Check sheet for the drawn part. Datum: minimum x, y, z corner. Units: mm. A direction names the side the tool comes from. Give positions to 0.01 mm unless a question says otherwise; leave off trailing zeros. Loops run counter-clockwise (first coordinate to the right, second up) from the corner with the lowest first, then second, coordinate; pieces in that order, holes last.
1. Cross-section at D-D, the plane x = 0.8. Record the cut outline in (y, z) (1 decimal).
2. Cross-section at B-B, the plane y = 6.75. Record the cut outline in (x, z) (1 decimal).
3. Tool access check on the marked faces 1, 2 and 3. Record the directions out of +Z, -Z, +X, -X, +Y, -Y that give a thin tool (end or side, any length) a straight path to the whole face; none if there is none.
4. Cross-section at C-C, the plane z = 13.75. Record the cut outline in (x, y).
5. Material ranges on L1, parallel to Z at x = 1.1, y = 11.5; L2, parallel to Z at x = 3.9, y = 12.25 (1 decimal); L3, parallel to Z at x = 1.2, y = 3, recorded low to high.
6. Go/stop test with flat-tipped pins: pin 1 Ø2 at (y, z) = (5, 9.5) entering from -X; pin 2 Ø1.7 at (y, z) = (2.159, 19.685) entering from -X; pin 3 Ø1.6 at (x, y) = (4, 9.5) entering from +Z (3 decimals); pin 4 Ø2.5 at (x, z) = (3.5, 11) entering from -Y. Record where each tip stops, or that it passes through.
7. Cross-section at A-A, the plane z = 2.5. Record the cut outline in (x, y) (1 decimal).
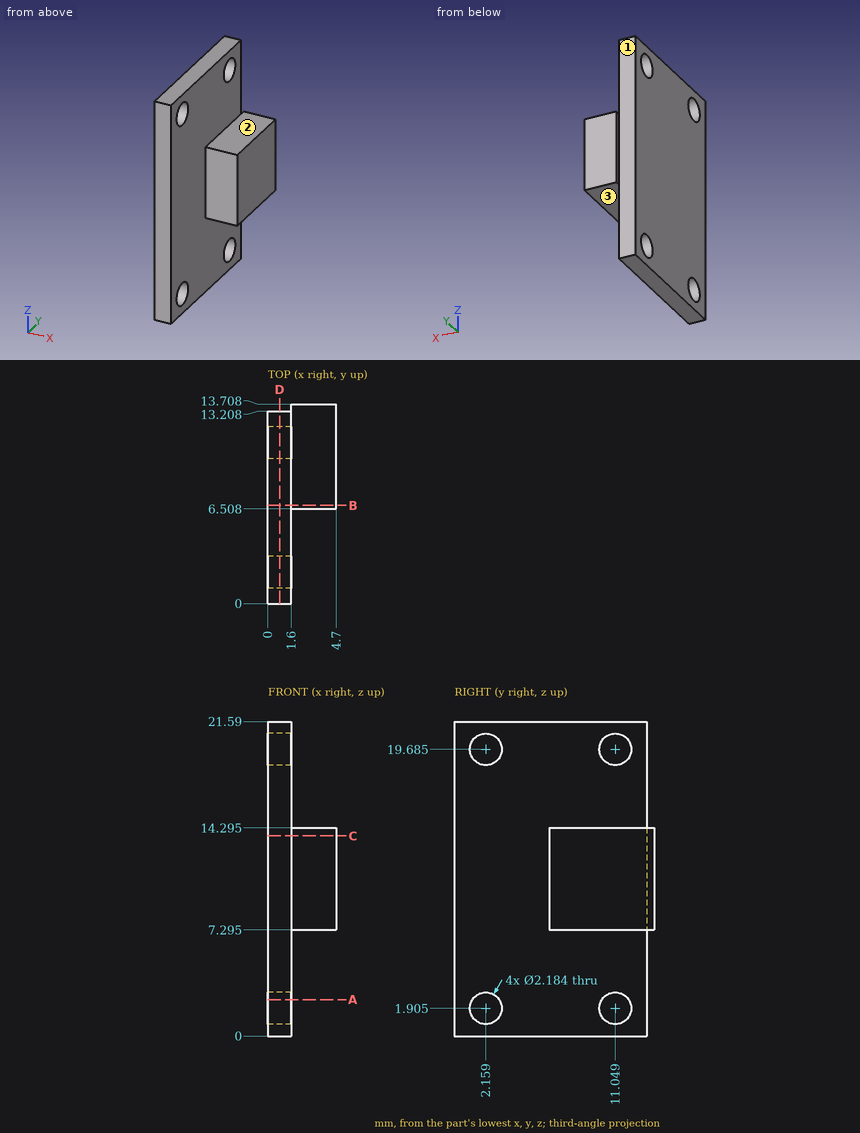
Result:
1. outline: (0, 0) - (13.2, 0) - (13.2, 21.6) - (0, 21.6) - close; hole circle Ø2.2 at (2.2, 1.9); hole circle Ø2.2 at (2.2, 19.7); hole circle Ø2.2 at (11, 1.9); hole circle Ø2.2 at (11, 19.7)
2. outline: (0, 0) - (1.6, 0) - (1.6, 7.3) - (4.7, 7.3) - (4.7, 14.3) - (1.6, 14.3) - (1.6, 21.6) - (0, 21.6) - close
3. face 1: +Z, -Z, -X, +Y
3. face 2: +Z, +X, +Y, -Y
3. face 3: -Z, +X, +Y, -Y
4. outline: (0, 0) - (1.6, 0) - (1.6, 6.51) - (4.7, 6.51) - (4.7, 13.71) - (1.6, 13.71) - (1.6, 13.21) - (0, 13.21) - close
5. L1: z = 0 to 0.91, 2.9 to 18.69, 20.68 to 21.59
5. L2: z = 7.3 to 14.3
5. L3: z = 0 to 1.21, 2.6 to 18.99, 20.38 to 21.59
6. pin 1: stops at x = 0
6. pin 2: passes through
6. pin 3: stops at z = 14.295
6. pin 4: stops at y = 6.51
7. outline: (0, 0) - (1.6, 0) - (1.6, 1.2) - (0, 1.2) - close; (0, 3.1) - (1.6, 3.1) - (1.6, 10.1) - (0, 10.1) - close; (0, 12) - (1.6, 12) - (1.6, 13.2) - (0, 13.2) - close
